```python
from build123d import *

# Parameters (mm, degrees)
SCHIZZO1_R                   = 135
ESTRUSIONE_ESTRUSIONE1_DEPTH = 5
SCHIZZO2_R                   = 115
TAGLIO_ESTRUSIONE1_DEPTH     = 191.984292548
SCHIZZO3_R                   = 2
ESTRUSIONE_ESTRUSIONE2_DEPTH = 3
RIPETIZIONECIRCOLARE1_COUNT  = 4
TAGLIO_ESTRUSIONE2_DEPTH     = 10
RIPETIZIONECIRCOLARE2_COUNT  = 4
TAGLIO_ESTRUSIONE21_DEPTH    = 8
RIPETIZIONECIRCOLARE3_COUNT  = 4
TAGLIO_ESTRUSIONE23_DEPTH    = 10
RIPETIZIONECIRCOLARE5_COUNT  = 4
RACCORDO1_R                  = 4
RACCORDO2_R                  = 4


with BuildPart() as part:
    # Schizzo1 → Estrusione-Estrusione1 (new body)
    with BuildSketch(Plane.XY):
        Circle(SCHIZZO1_R)
    extrude(amount=ESTRUSIONE_ESTRUSIONE1_DEPTH)

    # Schizzo2 → Taglio-Estrusione1 (cut, through all)
    with BuildSketch(Plane.XY.offset(5)):
        Circle(SCHIZZO2_R)
    extrude(amount=-TAGLIO_ESTRUSIONE1_DEPTH, mode=Mode.SUBTRACT)

    # Schizzo3 → Estrusione-Estrusione2 (add)
    with BuildSketch(Plane.XY.offset(5)):
        with Locations((0, 120)):
            Circle(SCHIZZO3_R)
    estrusione_estrusione2 = extrude(amount=ESTRUSIONE_ESTRUSIONE2_DEPTH)

    # RipetizioneCircolare1: Estrusione-Estrusione2 ×4 about axis
    ripetizionecircolare1_axis = Axis((0, 0, 0), (0, 0, 1))
    for i in range(1, RIPETIZIONECIRCOLARE1_COUNT):
        add(estrusione_estrusione2.rotate(ripetizionecircolare1_axis, i * 360 / RIPETIZIONECIRCOLARE1_COUNT))

    # Schizzo5 → Taglio-Estrusione2 (cut)
    with BuildSketch(Plane.XY.offset(5)):
        with BuildLine():
            ThreePointArc((-101.785752557, -75.95169897), (-56.934761924, -113.522829795), (0, -127))
            ThreePointArc((0, -127), (2, -125), (0, -123))
            ThreePointArc((0, -123), (-55.141541076, -109.947307596), (-98.579902083, -73.559519475))
            ThreePointArc((-98.579902083, -73.559519475), (-101.378917067, -73.152683985), (-101.785752557, -75.95169897))
        make_face()
    taglio_estrusione2 = extrude(amount=-TAGLIO_ESTRUSIONE2_DEPTH, mode=Mode.SUBTRACT)

    # RipetizioneCircolare2: Taglio-Estrusione2 ×4 about axis
    ripetizionecircolare2_axis = Axis((0, 0, 0), (0, 0, 1))
    for i in range(1, RIPETIZIONECIRCOLARE2_COUNT):
        add(taglio_estrusione2.rotate(ripetizionecircolare2_axis, i * 360 / RIPETIZIONECIRCOLARE2_COUNT), mode=Mode.SUBTRACT)

    # Schizzo14 → Taglio-Estrusione21 (cut)
    with BuildSketch(Plane.XY):
        Polygon((-39.736129967, 116.548444757), (-45.359906326, 140.907696377), (-21.000654706, 146.531472735), (-15.376878347, 122.172221115), align=None)
    taglio_estrusione21 = extrude(amount=TAGLIO_ESTRUSIONE21_DEPTH, mode=Mode.SUBTRACT)

    # RipetizioneCircolare3: Taglio-Estrusione21 ×4 about axis
    ripetizionecircolare3_axis = Axis((0, 0, 0), (0, 0, 1))
    for i in range(1, RIPETIZIONECIRCOLARE3_COUNT):
        add(taglio_estrusione21.rotate(ripetizionecircolare3_axis, i * 360 / RIPETIZIONECIRCOLARE3_COUNT), mode=Mode.SUBTRACT)

    # Schizzo15 → Taglio-Estrusione23 (cut)
    with BuildSketch(Plane.XY.offset(5)):
        with BuildLine():
            Line((-86.974134086, 86.974134086), (-81.317279836, 81.317279836))
            ThreePointArc((-81.317279836, 81.317279836), (-104.225395509, 48.6011001), (-114.562390281, 10.022910416))
            Line((-114.562390281, 10.022910416), (-122.531947865, 10.720156358))
            ThreePointArc((-122.531947865, 10.720156358), (-111.475857806, 51.982046194), (-86.974134086, 86.974134086))
        make_face()
    taglio_estrusione23 = extrude(amount=-TAGLIO_ESTRUSIONE23_DEPTH, mode=Mode.SUBTRACT)

    # RipetizioneCircolare5: Taglio-Estrusione23 ×4 about axis
    ripetizionecircolare5_axis = Axis((0, 0, 5), (0, 0, 1))
    for i in range(1, RIPETIZIONECIRCOLARE5_COUNT):
        add(taglio_estrusione23.rotate(ripetizionecircolare5_axis, i * 360 / RIPETIZIONECIRCOLARE5_COUNT), mode=Mode.SUBTRACT)

    # Raccordo1
    raccordo1_edges = [part.edges().sort_by_distance(p)[0] for p in [
        (-114.562390281, 10.022910416, 2.5),
        (-122.531947865, 10.720156358, 2.5),
    ]]
    fillet(raccordo1_edges, radius=RACCORDO1_R - 0.0001)  # a hair under: the kernel refuses the full size

    # Raccordo2
    raccordo2_edges = [part.edges().sort_by_distance(p)[0] for p in [
        (-81.317279836, -81.317279836, 2.5),
        (-86.974134086, -86.974134086, 2.5),
        (-10.022910416, -114.562390281, 2.5),
        (-10.720156358, -122.531947865, 2.5),
        (86.974134086, -86.974134086, 2.5),
        (81.317279836, -81.317279836, 2.5),
        (114.562390281, -10.022910416, 2.5),
        (122.531947865, -10.720156358, 2.5),
        (86.974134086, 86.974134086, 2.5),
        (81.317279836, 81.317279836, 2.5),
        (10.720156358, 122.531947865, 2.5),
        (10.022910416, 114.562390281, 2.5),
        (-81.317279836, 81.317279836, 2.5),
        (-86.974134086, 86.974134086, 2.5),
    ]]
    fillet(raccordo2_edges, radius=RACCORDO2_R - 0.0001)  # a hair under: the kernel refuses the full size


solid = part.part
```
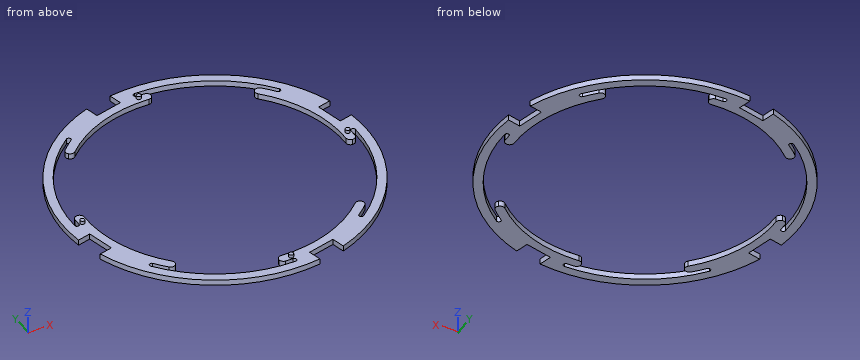
For this review, take the finished solid that the model builds, in its own axes (mm). Coordinates: 2 decimals unless noted, no trailing zeros. Order: outer loops, then holes, each group sorted by start corner. A loop starts at its lowest first (then second) coordinate and runs counter-clockwise, first axis right, second up. Notation, with made-up numbers: (3, 60.5) - (17, 60.5) arc R14 cw to (17, 78.5) - close; hole circle Ø7 at (51, 6). An arc over 180 degrees is marked (long way). Answer as a JSON object with one key per item and string values. Group by question number.
1. We need section A-A on y = -52. State the section outline as (x, z) points, then the cut area to 3 significant figures.
2. For probe 1 along X at (y, z) = (7, 2.25); probe 2 along X at (y, z) = (102, 0.5); probe 3 along Z at (x, y) = (69.5, -110.5), list the stretches that pass through material, from the lowest coordinate up.
3. Clearance check with flat-ended pins moving along their axes: P1, Ø2, axis at y = -79, z = 5.5, coming from the +X side; P2, Ø4, axis at y = -9, z = 6.5, coming from the -X side. State where each tip first meets the part, or that it passes through.
Final values:
{
 "1": {"outline": "(-124.58, 0) - (-102.57, 0) - (-102.57, 5) - (-124.58, 5) - close; (115.87, 0) - (124.58, 0) - (124.58, 5) - (115.87, 5) - close", "area": "154 mm²"},
 "2": {"probe 1": "-134.82 to -126.81, -122.78 to -114.88, 114.79 to 134.82", "probe 2": "-88.44 to -75.59, -73.92 to -53.11, 75.66 to 88.44", "probe 3": "0 to 5"},
 "3": {"P1": "x = 110.09", "P2": "x = -134.78"}
}
